from build123d import *
from build123d.topology import SkipClean

# Parameters (mm, degrees)
BOSS_EXTRUDE1_DEPTH     = 12
SKETCH3_R               = 1.8
CUT_EXTRUDE2_DEPTH      = 13
CUT_EXTRUDE2_DEPTH_BACK = 1
BOSS_EXTRUDE2_DEPTH     = 3
CUT_EXTRUDE4_DEPTH      = 16
SKETCH7_R               = 2.8
SKETCH7_R_2             = 1.8
BOSS_EXTRUDE3_DEPTH     = 8


with BuildPart() as part:
    # Sketch1 → Boss-Extrude1 (new body)
    with BuildSketch(Plane.XY):
        with BuildLine():
            Line((0, 12.5), (16.2, 12.5))
            ThreePointArc((16.2, 12.5), (8.1, -2.790812019), (0, 12.5))
        make_face()
    extrude(amount=BOSS_EXTRUDE1_DEPTH)

    # Sketch3 → Cut-Extrude2 (cut, two sides)
    with BuildSketch(Plane.XY) as cut_extrude2_sk:
        with Locations((8.1, 7)):
            Circle(SKETCH3_R)
    extrude(amount=CUT_EXTRUDE2_DEPTH, mode=Mode.SUBTRACT)
    extrude(cut_extrude2_sk.sketch, amount=-CUT_EXTRUDE2_DEPTH_BACK, mode=Mode.SUBTRACT)

    # Sketch4 → Boss-Extrude2 (add)
    with SkipClean():  # the faces are left unmerged after this step: merging them gives an invalid solid
        with BuildSketch(Plane.XY):
            with BuildLine():
                Line((16.2, 12.5), (15.362063339, 12.5))
                ThreePointArc((15.362063339, 12.5), (14.070641831, 11.763040292), (14.048187812, 10.276307316))
                ThreePointArc((14.048187812, 10.276307316), (8.1, 0.209187981), (2.151812188, 10.276307316))
                ThreePointArc((2.151812188, 10.276307316), (2.129358169, 11.763040292), (0.837936661, 12.5))
                Line((0.837936661, 12.5), (0, 12.5))
                ThreePointArc((0, 12.5), (8.1, -2.790812019), (16.2, 12.5))
            make_face()
        extrude(amount=-BOSS_EXTRUDE2_DEPTH)

    # Sketch6 → Cut-Extrude4 (cut)
    with SkipClean():  # the faces are left unmerged after this step: merging them gives an invalid solid
        with BuildSketch(Plane(origin=(0.1, 0, 0), x_dir=(0, 0, -1), z_dir=(1, 0, 0))):
            with BuildLine():
                Line((-9, 2.60459399), (-4, 2.60459399))
                Line((-4, 2.60459399), (-4, 12.5))
                Line((-4, 12.5), (-8.5, 12.5))
                Line((-8.5, 12.5), (-8.5, 7.10459399))
                Line((-8.5, 7.10459399), (-9, 7.10459399))
                ThreePointArc((-9, 7.10459399), (-11.25, 4.85459399), (-9, 2.60459399))
            make_face()
        extrude(amount=CUT_EXTRUDE4_DEPTH, mode=Mode.SUBTRACT)

    # Sketch7 → Boss-Extrude3 (add)
    with SkipClean():  # the faces are left unmerged after this step: merging them gives an invalid solid
        with BuildSketch(Plane.XY.offset(4)):
            with Locations(Location((8.1, 7, 0), (0, 0, 177.859218285))):
                Circle(SKETCH7_R)
            with Locations((8.1, 7)):
                Circle(SKETCH7_R_2, mode=Mode.SUBTRACT)
        extrude(amount=BOSS_EXTRUDE3_DEPTH)


solid = part.part
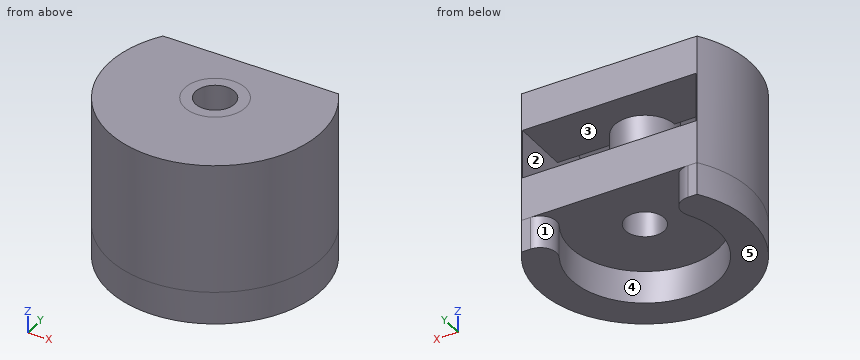
Could you check a few things on this model? Use its own coordinates, in mm. Face numbers are marked on the shaded views. A direction names the side the tool comes from. Give positions to 0.01 mm unless a question says otherwise; leave off trailing zeros. Order: outer loops, then holes, each group sorted by start corner. A loop starts at its lowest first (then second) coordinate and runs counter-clockwise, first axis right, second up.
Item 1: If we section it at A-A, the plane z = 6.25: Write out the boundary of the cut face in (x, y), plus the area to 3 significant figures.
Item 2: I'm going to push flat-ended pins straight in: pin 1 (1.5 mm diameter, centred on y = 4, z = 9, fed in from +X); pin 2 (3 mm diameter, centred on x = 8.1, y = 7, fed in from -Z); pin 3 (1.5 mm diameter, centred on y = 8, z = 6, fed in from +X); pin 4 (2 mm diameter, centred on y = 3.5, z = 4.5, fed in from -X). Where does each tip first touch, or does it pass through?
Item 3: If we section it at B-B, the plane x = 9: Write out the boundary of the cut face in (y, z), plus the area to 3 significant figures.
Item 4: If we mould it in two halves opening along X, with no side actions, what happens to the marked faces 4 and 5? For each: pulls with the +X half, pulls with the -X half, needs draft (parallel to the pull), parting line crosses it, or undercut.
Item 5: For the marked faces 1, 2 and 3, which set-ups out of +Z, -Z, +X, -X, +Y, -Y let a thin tool reach every point of the face, with its end or its side?
Item 6: If we section it at D-D, the plane y = 3.75: Write out the boundary of the cut face in (x, z), plus the area to 3 significant figures.
Item 7: I need wall thicknesses on line 1 (X direction, y = 7, z = 7.25); line 2 (Z direction, x = 0.5, y = 8.5); line 3 (Z direction, x = 0.5, y = 4.75). Which ranges of each line are inside material? Lowest first, please.
Item 8: If we section it at C-C, the plane y = 7.75: Write out the boundary of the cut face in (x, z).
Values:
1. outline: (0, 12.5) arc R9.79 ccw (long way) to (16.2, 12.5) - (16.1, 12.5) - (16.1, 2.6) - (0.1, 2.6) - (0.1, 12.5) - close; circle Ø5.6 at (8.1, 7); hole circle Ø3.6 at (8.1, 7)
1. area: 108 mm2
2. pin 1: stops at x = 17.63
2. pin 2: passes through
2. pin 3: stops at x = 17.89
2. pin 4: stops at x = -1.37
3. outline: (-2.75, -3) - (0.27, -3) - (0.27, 0) - (5.44, 0) - (5.44, 12) - (-2.75, 12) - close; (8.56, 0) - (12.5, 0) - (12.5, 4) - (9.65, 4) - (9.65, 8.5) - (12.5, 8.5) - (12.5, 12) - (8.56, 12) - close; hole (2.6, 4) - (4.35, 4) - (4.35, 11.19) arc R2.25 ccw to (2.6, 9) - close
3. area: 130 mm2
4. face 4: undercut
4. face 5: needs draft
5. face 1: -Z
5. face 2: none
5. face 3: +Y
6. outline: (-1.14, -3) - (2.14, -3) - (2.14, 0) - (14.06, 0) - (14.06, -3) - (17.34, -3) - (17.34, 12) - (-1.14, 12) - close; hole (0.1, 4) - (16.1, 4) - (16.1, 10.96) - (0.1, 10.96) - close
6. area: 130 mm2
7. line 1: x = -1.69 to 0.1, 5.3 to 6.3, 9.9 to 10.9, 16.1 to 17.89
7. line 2: z = -3 to 4, 8.5 to 12
7. line 3: z = -3 to 4, 11.25 to 12
8. outline: (-1.66, -3) - (1.35, -3) - (1.35, 0) - (6.46, 0) - (6.46, 12) - (-1.66, 12) - close; (9.74, 0) - (14.85, 0) - (14.85, -3) - (17.86, -3) - (17.86, 12) - (9.74, 12) - close; hole (0.1, 4) - (5.4, 4) - (5.4, 8.5) - (0.1, 8.5) - close; hole (10.8, 4) - (16.1, 4) - (16.1, 8.5) - (10.8, 8.5) - close
